```python
from build123d import *

# Parameters (mm, degrees)
SKIZZE1_W                       = 164
SKIZZE1_H                       = 94
AUFSATZ_LINEAR_AUSTRAGEN1_DEPTH = 25
AUFSATZ_LINEAR_AUSTRAGEN2_DEPTH = 164
SCHNITT_LINEAR_AUSTRAGEN1_REACH = 106.68
AUFSATZ_LINEAR_AUSTRAGEN3_REACH = 106.68
SKIZZE4_R                       = 4.236153916
SKIZZE4_R_2                     = 1.5
SCHNITT_LINEAR_AUSTRAGEN2_DEPTH = 4.05
VERRUNDUNG1_R                   = 5
SKIZZE7_W                       = 9
SKIZZE7_H                       = 4
SCHNITT_LINEAR_AUSTRAGEN4_DEPTH = 4.05
SKIZZE8_R                       = 5.5
SCHNITT_LINEAR_AUSTRAGEN5_DEPTH = 1
SKIZZE9_W                       = 47.666626173
SKIZZE9_H                       = 143.1878039
SKIZZE9_W_2                     = 41.660611838
SCHNITT_LINEAR_AUSTRAGEN6_DEPTH = 105.680466182
SCHNITT_LINEAR_AUSTRAGEN7_REACH = 103.419


with BuildPart() as part:
    # Skizze1 → Aufsatz-Linear austragen1 (new body)
    with BuildSketch(Plane.XY):
        Rectangle(SKIZZE1_W, SKIZZE1_H)
    extrude(amount=AUFSATZ_LINEAR_AUSTRAGEN1_DEPTH)

    # Skizze2 → Aufsatz-Linear austragen2 (add)
    with BuildSketch(Plane(origin=(82, 0, 0), x_dir=(0, 0, -1), z_dir=(1, 0, 0))):
        Polygon((0, -47), (0, 47), (20, 47), align=None)
    extrude(amount=-AUFSATZ_LINEAR_AUSTRAGEN2_DEPTH)

    # Schnitt-Linear austragen1: up to this plane
    schnitt_linear_austragen1_end = Plane(origin=(-82, 47.416215289, -18.043788142), z_dir=(0, -0.20810764446485866, -0.9781059289848355))
    # Skizze3 → Schnitt-Linear austragen1 (cut, up to the surface)
    with BuildSketch(Plane.XY.offset(25), mode=Mode.PRIVATE) as schnitt_linear_austragen1_sk1:
        with BuildLine():
            Line((-75.15, -45.15), (75.15, -45.15))
            ThreePointArc((75.15, -45.15), (78.685533906, -43.685533906), (80.15, -40.15))
            Line((80.15, -40.15), (80.15, 40.15))
            ThreePointArc((80.15, 40.15), (78.685533906, 43.685533906), (75.15, 45.15))
            Line((75.15, 45.15), (-75.15, 45.15))
            ThreePointArc((-75.15, 45.15), (-78.685533906, 43.685533906), (-80.15, 40.15))
            Line((-80.15, 40.15), (-80.15, -40.15))
            ThreePointArc((-80.15, -40.15), (-78.685533906, -43.685533906), (-75.15, -45.15))
        make_face()
    schnitt_linear_austragen1_tool1 = split(extrude(schnitt_linear_austragen1_sk1.sketch, amount=-SCHNITT_LINEAR_AUSTRAGEN1_REACH, mode=Mode.PRIVATE), bisect_by=schnitt_linear_austragen1_end, keep=Keep.BOTH, mode=Mode.PRIVATE)
    add(schnitt_linear_austragen1_tool1.solids().sort_by_distance((0, 0, 25))[0], mode=Mode.SUBTRACT)

    # Aufsatz-Linear austragen3: up to this plane
    aufsatz_linear_austragen3_end = Plane(origin=(-82, 47.416215289, -18.043788142), z_dir=(0, -0.20810764446485866, -0.9781059289848355))
    # Skizze4 → Aufsatz-Linear austragen3 (add, up to the surface)
    with BuildSketch(Plane.XY.offset(25), mode=Mode.PRIVATE) as aufsatz_linear_austragen3_sk1:
        with Locations((-76, 41)):
            Circle(SKIZZE4_R)
        with Locations((-76, 41)):
            Circle(SKIZZE4_R_2, mode=Mode.SUBTRACT)
    aufsatz_linear_austragen3_tool1 = split(extrude(aufsatz_linear_austragen3_sk1.sketch, amount=-AUFSATZ_LINEAR_AUSTRAGEN3_REACH, mode=Mode.PRIVATE), bisect_by=aufsatz_linear_austragen3_end, keep=Keep.BOTH, mode=Mode.PRIVATE)
    add(aufsatz_linear_austragen3_tool1.solids().sort_by_distance((-80.116337, 41, 25))[0])
    # Skizze4 → Aufsatz-Linear austragen3 (add, up to the surface)
    with BuildSketch(Plane.XY.offset(25), mode=Mode.PRIVATE) as aufsatz_linear_austragen3_sk2:
        with Locations((-76, -41)):
            Circle(SKIZZE4_R)
        with Locations((-76, -41)):
            Circle(SKIZZE4_R_2, mode=Mode.SUBTRACT)
    aufsatz_linear_austragen3_tool2 = split(extrude(aufsatz_linear_austragen3_sk2.sketch, amount=-AUFSATZ_LINEAR_AUSTRAGEN3_REACH, mode=Mode.PRIVATE), bisect_by=aufsatz_linear_austragen3_end, keep=Keep.BOTH, mode=Mode.PRIVATE)
    add(aufsatz_linear_austragen3_tool2.solids().sort_by_distance((-80.116337, -41, 25))[0])
    # Skizze4 → Aufsatz-Linear austragen3 (add, up to the surface)
    with BuildSketch(Plane.XY.offset(25), mode=Mode.PRIVATE) as aufsatz_linear_austragen3_sk3:
        with Locations((76, -41)):
            Circle(SKIZZE4_R)
        with Locations((76, -41)):
            Circle(SKIZZE4_R_2, mode=Mode.SUBTRACT)
    aufsatz_linear_austragen3_tool3 = split(extrude(aufsatz_linear_austragen3_sk3.sketch, amount=-AUFSATZ_LINEAR_AUSTRAGEN3_REACH, mode=Mode.PRIVATE), bisect_by=aufsatz_linear_austragen3_end, keep=Keep.BOTH, mode=Mode.PRIVATE)
    add(aufsatz_linear_austragen3_tool3.solids().sort_by_distance((71.883663, -41, 25))[0])
    # Skizze4 → Aufsatz-Linear austragen3 (add, up to the surface)
    with BuildSketch(Plane.XY.offset(25), mode=Mode.PRIVATE) as aufsatz_linear_austragen3_sk4:
        with Locations((76, 41)):
            Circle(SKIZZE4_R)
        with Locations((76, 41)):
            Circle(SKIZZE4_R_2, mode=Mode.SUBTRACT)
    aufsatz_linear_austragen3_tool4 = split(extrude(aufsatz_linear_austragen3_sk4.sketch, amount=-AUFSATZ_LINEAR_AUSTRAGEN3_REACH, mode=Mode.PRIVATE), bisect_by=aufsatz_linear_austragen3_end, keep=Keep.BOTH, mode=Mode.PRIVATE)
    add(aufsatz_linear_austragen3_tool4.solids().sort_by_distance((71.883663, 41, 25))[0])

    # Skizze6 → Schnitt-Linear austragen2 (cut)
    with BuildSketch(Plane.XY.offset(25)):
        with BuildLine():
            Line((-75.15, -45.15), (75.15, -45.15))
            ThreePointArc((75.15, -45.15), (78.685533906, -43.685533906), (80.15, -40.15))
            Line((80.15, -40.15), (80.15, 40.15))
            ThreePointArc((80.15, 40.15), (78.685533906, 43.685533906), (75.15, 45.15))
            Line((75.15, 45.15), (-75.15, 45.15))
            ThreePointArc((-75.15, 45.15), (-78.685533906, 43.685533906), (-80.15, 40.15))
            Line((-80.15, 40.15), (-80.15, -40.15))
            ThreePointArc((-80.15, -40.15), (-78.685533906, -43.685533906), (-75.15, -45.15))
        make_face()
    extrude(amount=-SCHNITT_LINEAR_AUSTRAGEN2_DEPTH, mode=Mode.SUBTRACT)

    # Verrundung1
    verrundung1_edges = [part.edges().sort_by_distance(p)[0] for p in [
        (82, -47, 12.5),
        (-82, -47, 12.5),
        (-82, 47, 2.5),
        (82, 47, 2.5),
    ]]
    fillet(verrundung1_edges, radius=VERRUNDUNG1_R)

    # Skizze7 → Schnitt-Linear austragen4 (cut)
    with BuildSketch(Plane(origin=(0, 47, 0), x_dir=(1, 0, 0), z_dir=(0, 1, 0))):
        with Locations((13.5, 12.561614676)):
            Rectangle(SKIZZE7_W, SKIZZE7_H)
    extrude(amount=-SCHNITT_LINEAR_AUSTRAGEN4_DEPTH, mode=Mode.SUBTRACT)

    # Skizze8 → Schnitt-Linear austragen5 (cut)
    with BuildSketch(Plane(origin=(0, -2.035513209, -9.566912083), x_dir=(-1, 0, 0), z_dir=(0, -0.20810764446485866, -0.9781059289848355))):
        with Locations(Location((-72, 40.133131552, 0), (0, 0, 90))):
            Circle(SKIZZE8_R)
        with Locations(Location((72, 40.133131552, 0), (0, 0, 90))):
            Circle(SKIZZE8_R)
        with Locations(Location((72, -35.970978662, 0), (0, 0, 90))):
            Circle(SKIZZE8_R)
        with Locations(Location((-72, -35.970978662, 0), (0, 0, 90))):
            Circle(SKIZZE8_R)
    extrude(amount=-SCHNITT_LINEAR_AUSTRAGEN5_DEPTH, mode=Mode.SUBTRACT)

    # Skizze9 → Schnitt-Linear austragen6 (cut, through all)
    with BuildSketch(Plane.XY.offset(25)):
        with Locations((103.833313086, 0)):
            Rectangle(SKIZZE9_W, SKIZZE9_H)
        with Locations((-100.830305919, 0)):
            Rectangle(SKIZZE9_W_2, SKIZZE9_H)
    extrude(amount=-SCHNITT_LINEAR_AUSTRAGEN6_DEPTH, mode=Mode.SUBTRACT)

    # Schnitt-Linear austragen7: up to this plane
    schnitt_linear_austragen7_end = Plane(origin=(-82, 47.416215289, -18.043788142), z_dir=(0, -0.20810764446485866, -0.9781059289848355))
    # Skizze11 → Schnitt-Linear austragen7 (cut, up to the surface)
    with BuildSketch(Plane.XY.offset(20.95), mode=Mode.PRIVATE) as schnitt_linear_austragen7_sk1:
        Polygon((-77.9, 43), (-79, 43), (-79, 40.1), (-80, 40.1), (-80, -40.1), (-79, -40.1), (-79, -43), (-77.9, -43), align=None)
    schnitt_linear_austragen7_tool1 = split(extrude(schnitt_linear_austragen7_sk1.sketch, amount=-SCHNITT_LINEAR_AUSTRAGEN7_REACH, mode=Mode.PRIVATE), bisect_by=schnitt_linear_austragen7_end, keep=Keep.BOTH, mode=Mode.PRIVATE)
    add(schnitt_linear_austragen7_tool1.solids().sort_by_distance((-78.931751, 0, 20.95))[0], mode=Mode.SUBTRACT)
    # Skizze11 → Schnitt-Linear austragen7 (cut, up to the surface)
    with BuildSketch(Plane.XY.offset(20.95), mode=Mode.PRIVATE) as schnitt_linear_austragen7_sk2:
        Polygon((80, 40.1), (80, -40.1), (79, -40.1), (79, -43), (77.9, -43), (77.9, 43), (79, 43), (79, 40.1), align=None)
    schnitt_linear_austragen7_tool2 = split(extrude(schnitt_linear_austragen7_sk2.sketch, amount=-SCHNITT_LINEAR_AUSTRAGEN7_REACH, mode=Mode.PRIVATE), bisect_by=schnitt_linear_austragen7_end, keep=Keep.BOTH, mode=Mode.PRIVATE)
    add(schnitt_linear_austragen7_tool2.solids().sort_by_distance((78.931751, 0, 20.95))[0], mode=Mode.SUBTRACT)


solid = part.part
```
Model file for the job. Use its own axes, mm. A direction names the side the tool comes from. Give positions to 0.01 mm unless a question says otherwise; leave off trailing zeros. Write each loop counter-clockwise with the first axis right and the second up, starting at its lowest first coordinate (ties: lowest second). Pieces come first, ordered by that corner, then holes. Notation, with made-up numbers: M 6,-38.5 L 60,-38.5 A24 ccw 60,-20.5 Z; hole C 69.5,-23.5 d9. An arc over 180 degrees is marked long. Use a Markdown table: item, result.
1) Drill centre lines: line 1 (X direction, y = 41, z = 7.5); line 2 (Y direction, x = 76, z = 6); line 3 (Y direction, x = 7, z = 15). Where is each one in solid material? Low to high. Write a range as from..to.
Responses:
| item | result |
|---|---|
| line 1 | x = -80..-79, -77.9..-77.5, -74.5..-71.76, 71.76..74.5, 77.5..77.9, 79..80 |
| line 2 | y = -47..-42.5, -39.5..-36.76, 36.76..39.5, 42.5..47 |
| line 3 | y = -47..-45.15, 45.15..47 |
2) Cut at A-A (z = -6). List the corners of the cut face in (x, y).
Responses:
| item | result |
|---|---|
| outline | M -80,-18.8 L 80,-18.8 L 80,-9.19 L -80,-9.19 Z; M -80,40.1 L -79,40.1 L -79,43 L -77.9,43 L -77.9,37.21 A4.24 ccw long -75.15,45.15 L 75.15,45.15 A4.24 ccw long 77.9,37.21 L 77.9,43 L 79,43 L 79,40.1 L 80,40.1 L 80,46 A5 ccw 77,47 L -77,47 A5 ccw -80,46 Z; hole C -76,41 d3; hole C 76,41 d3 |
3) Pin check, flat tips, straight feed: pin 1 (5 mm diameter, centred on y = 5, z = -8, fed in from +X); pin 2 (9 mm diameter, centred on x = -74.5, y = 40.5, fed in from +Z); pin 3 (6 mm diameter, centred on x = -12, y = 23, fed in from +Z); pin 4 (0.9 mm diameter, centred on x = -78.5, z = 9.5, fed in from +Y). Stop position of each tip, or through.
Responses:
| item | result |
|---|---|
| pin 1 | stops at x = 80 |
| pin 2 | stops at z = 20.95 |
| pin 3 | stops at z = -12.21 |
| pin 4 | stops at y = 46.89 |
4) Cut at C-C (x = -28). List the corners of the cut face in (y, z), and give its area (3 significant figures).
Responses:
| item | result |
|---|---|
| outline | M -47,0 L 47,-20 L 47,25 L 45.15,25 L 45.15,-17.56 L -45.15,1.65 L -45.15,25 L -47,25 Z |
| area | 314 mm2 |
5) Tool access for faces 1 (the flat face through (-77.9, -40, 11)), 2 (the flat face through (80, 3, -9)): list every direction of +Z, -Z, +X, -X, +Y, -Y with a clear straight run to the whole face (end or side of a thin tool).
Responses:
| item | result |
|---|---|
| face 1 | +Z |
| face 2 | +Z, -Z, +X, +Y, -Y |
6) Cut at D-D (y = -8). List the corners of the cut face in (x, z), and give its area (3 significant figures).
Responses:
| item | result |
|---|---|
| outline | M -80,-8.3 L 80,-8.3 L 80,-6.25 L -80,-6.25 Z |
| area | 327 mm2 |
7) Cut at B-B (z = 22.5). List the corners of the cut face in (x, y).
Responses:
| item | result |
|---|---|
| outline | M -80,-46 A5 ccw -77,-47 L 77,-47 A5 ccw 80,-46 L 80,-41.37 A5 cw 75.15,-45.15 L -75.15,-45.15 A5 cw -80,-41.37 Z; M -80,41.37 A5 cw -75.15,45.15 L 75.15,45.15 A5 cw 80,41.37 L 80,46 A5 ccw 77,47 L -77,47 A5 ccw -80,46 Z |
8) Pull direction Z, two halves, no side cores. Call faces 3 (the flat face through (77.9, -40, 11)), 4 (the cylindrical face through (77.453, -37.817, -1.45)), 5 (the cylindrical face through (-66.547, 36.621, -17.288)), 6 (the flat face through (74, -41, 20.95)): +Z half, -Z half, draft (parallel to the pull), parting line (faces both ways), or undercut.
Responses:
| item | result |
|---|---|
| face 3 | draft |
| face 4 | undercut |
| face 5 | undercut |
| face 6 | +Z half |
